Drawing for the job (mm, zero at the part's lowest x, y, z). A direction names the side the tool comes from. Coordinates: 2 decimals unless noted, no trailing zeros. Write each loop counter-clockwise with the first axis right and the second up, starting at its lowest first coordinate (ties: lowest second). Pieces come first, ordered by that corner, then holes. Notation, with made-up numbers: (22, -30.5) -> (65, -30.5) arc R18 ccw to (65, -12.5) -> close; hole circle Ø4 at (51.5, 62). An arc over 180 degrees is marked (long way). Answer as CSV lines item,"result".
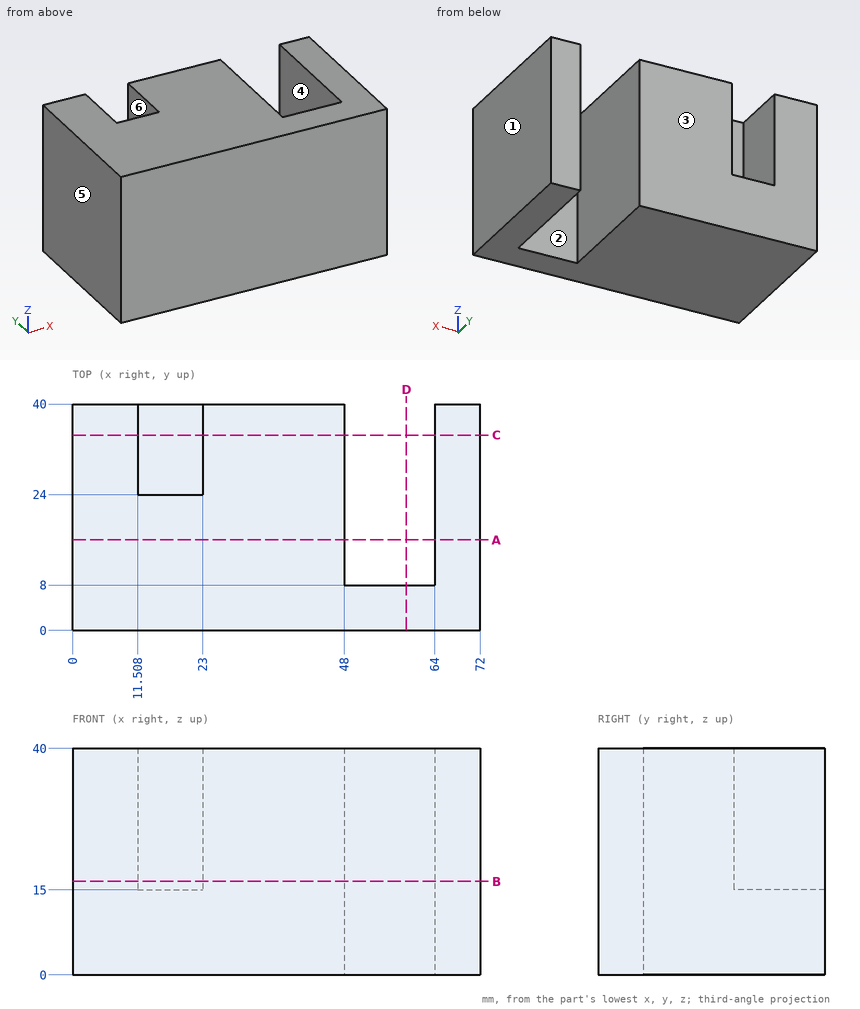
Item 1: Saw through at D-D on x = 59. Give the cut face in (y, z).
Answer below:
outline,"(0, 0) -> (8, 0) -> (8, 40) -> (0, 40) -> close"
Item 2: Two-plate mould, pull along X, no slides. Class the marked faces 1, 2 and 3: pulls with the +X half, pulls with the -X half, needs draft (parallel to the pull), parting line crosses it, or undercut.
Answer below:
face 1,"pulls with the +X half"
face 2,"undercut"
face 3,"needs draft"
Item 3: Saw through at B-B on z = 16.5. Give the cut face in (x, y), and give its area (3 significant figures).
Answer below:
outline,"(0, 0) -> (72, 0) -> (72, 40) -> (64, 40) -> (64, 8) -> (48, 8) -> (48, 40) -> (23, 40) -> (23, 24) -> (11.51, 24) -> (11.51, 40) -> (0, 40) -> close"
area,"2,180 mm2"
Item 4: Flat gauge pin, fed straight in: pin 1 (9 mm diameter, centred on x = 18, z = 28.5, fed in from +Y). Where does the tip first touch, or does it go through?
Answer below:
pin 1,"stops at y = 24"
Item 5: 3-axis set-ups, long thin cutter, end or side, ignore diameter. For the marked faces 4, 5 and 6: which of +Z, -Z, +X, -X, +Y, -Y reach the whole face in a straight line?
Answer below:
face 4,"+Z, -Z, +Y"
face 5,"+Z, -Z, -X, +Y, -Y"
face 6,"+Z, +Y"
Item 6: Saw through at A-A on y = 16. Give the cut face in (x, z).
Answer below:
outline,"(0, 0) -> (48, 0) -> (48, 40) -> (0, 40) -> close; (64, 0) -> (72, 0) -> (72, 40) -> (64, 40) -> close"
Item 7: Wall check: line 1 (X direction, y = 35.5, z = 28); line 2 (X direction, y = 10, z = 5.5); line 3 (Y direction, x = 61.5, z = 28). Give the ranges that are in metal, low to high. Write a range as from..to.
Answer below:
line 1,"x = 0..11.51, 23..48, 64..72"
line 2,"x = 0..48, 64..72"
line 3,"y = 0..8"
Item 8: Saw through at C-C on y = 34.5. Give the cut face in (x, z).
Answer below:
outline,"(0, 0) -> (48, 0) -> (48, 40) -> (23, 40) -> (23, 15) -> (11.51, 15) -> (11.51, 40) -> (0, 40) -> close; (64, 0) -> (72, 0) -> (72, 40) -> (64, 40) -> close"
